from build123d import *

# Parameters (mm, degrees)
SKETCH1_R                 = 13
BOSS_EXTRUDE1_DEPTH       = 65
BOSS_EXTRUDE1_DEPTH_BACK  = 65
SKETCH6_R                 = 2.5
BOSS_EXTRUDE5_DEPTH       = 35
SKETCH7_R                 = 2.5
BOSS_EXTRUDE6_DEPTH       = 35
SKETCH10_R                = 2.5
BOSS_EXTRUDE7_DEPTH       = 20
BOSS_EXTRUDE7_DEPTH_BACK  = 20
SKETCH11_R                = 2.5
BOSS_EXTRUDE8_DEPTH       = 45
SKETCH12_W                = 11.53
SKETCH12_H                = 5
BOSS_EXTRUDE9_DEPTH       = 12
SKETCH13_R                = 4.765
CUT_EXTRUDE2_DEPTH        = 66
CUT_EXTRUDE2_DEPTH_BACK   = 12
SKETCH14_R                = 2.5
BOSS_EXTRUDE10_DEPTH      = 20
BOSS_EXTRUDE10_DEPTH_BACK = 20
SKETCH15_R                = 2.5
BOSS_EXTRUDE11_DEPTH      = 45
SKETCH16_W                = 11.53
SKETCH16_H                = 5
BOSS_EXTRUDE12_DEPTH      = 12
SKETCH17_R                = 4.765
CUT_EXTRUDE3_DEPTH        = 12
CUT_EXTRUDE3_DEPTH_BACK   = 51


with BuildPart() as part:
    # Sketch1 → Boss-Extrude1 (new body, two sides)
    with BuildSketch(Plane(origin=(0, 0, 0), x_dir=(0, 0, -1), z_dir=(1, 0, 0))) as boss_extrude1_sk:
        Circle(SKETCH1_R)
    extrude(amount=BOSS_EXTRUDE1_DEPTH)
    extrude(boss_extrude1_sk.sketch, amount=-BOSS_EXTRUDE1_DEPTH_BACK)

    # Sketch6 → Boss-Extrude5 (add)
    with BuildSketch(Plane(origin=(65, 0, 0), x_dir=(0, 0, -1), z_dir=(1, 0, 0))):
        Circle(SKETCH6_R)
    extrude(amount=BOSS_EXTRUDE5_DEPTH)

    # Sketch7 → Boss-Extrude6 (add)
    with BuildSketch(Plane.ZY.offset(65)):
        Circle(SKETCH7_R)
    extrude(amount=BOSS_EXTRUDE6_DEPTH)

    # Sketch10 → Boss-Extrude7 (add, two sides)
    with BuildSketch(Plane.YX) as boss_extrude7_sk:
        with Locations((0, 100)):
            Circle(SKETCH10_R)
    extrude(amount=BOSS_EXTRUDE7_DEPTH)
    extrude(boss_extrude7_sk.sketch, amount=-BOSS_EXTRUDE7_DEPTH_BACK)

    # Sketch11 → Boss-Extrude8 (add)
    with BuildSketch(Plane(origin=(0, 0, 0), x_dir=(1, 0, 0), z_dir=(0, 1, 0))):
        with Locations((100, -20)):
            Circle(SKETCH11_R)
        with Locations((100, 20)):
            Circle(SKETCH11_R)
    extrude(amount=BOSS_EXTRUDE8_DEPTH)

    # Sketch12 → Boss-Extrude9 (add)
    with BuildSketch(Plane(origin=(0, 45, 0), x_dir=(1, 0, 0), z_dir=(0, 1, 0))):
        with Locations((100, -20)):
            Rectangle(SKETCH12_W, SKETCH12_H)
        with Locations((100, 20)):
            Rectangle(SKETCH12_W, SKETCH12_H)
    extrude(amount=BOSS_EXTRUDE9_DEPTH)

    # Sketch13 → Cut-Extrude2 (cut, two sides)
    with BuildSketch(Plane.XY.offset(-17.5)) as cut_extrude2_sk:
        with Locations((100.265, 51)):
            Circle(SKETCH13_R)
    extrude(amount=CUT_EXTRUDE2_DEPTH, mode=Mode.SUBTRACT)
    extrude(cut_extrude2_sk.sketch, amount=-CUT_EXTRUDE2_DEPTH_BACK, mode=Mode.SUBTRACT)

    # Sketch14 → Boss-Extrude10 (add, two sides)
    with BuildSketch(Plane.XY) as boss_extrude10_sk:
        with Locations((-100, 0)):
            Circle(SKETCH14_R)
    extrude(amount=BOSS_EXTRUDE10_DEPTH)
    extrude(boss_extrude10_sk.sketch, amount=-BOSS_EXTRUDE10_DEPTH_BACK)

    # Sketch15 → Boss-Extrude11 (add)
    with BuildSketch(Plane(origin=(0, 0, 0), x_dir=(1, 0, 0), z_dir=(0, 1, 0))):
        with Locations((-100, 20)):
            Circle(SKETCH15_R)
        with Locations((-100, -20)):
            Circle(SKETCH15_R)
    extrude(amount=BOSS_EXTRUDE11_DEPTH)

    # Sketch16 → Boss-Extrude12 (add)
    with BuildSketch(Plane(origin=(0, 45, 0), x_dir=(1, 0, 0), z_dir=(0, 1, 0))):
        with Locations((-100, -20)):
            Rectangle(SKETCH16_W, SKETCH16_H)
        with Locations((-100, 20)):
            Rectangle(SKETCH16_W, SKETCH16_H)
    extrude(amount=BOSS_EXTRUDE12_DEPTH)

    # Sketch17 → Cut-Extrude3 (cut, two sides)
    with BuildSketch(Plane.XY.offset(22.5)) as cut_extrude3_sk:
        with Locations((-99.735, 51)):
            Circle(SKETCH17_R)
    extrude(amount=CUT_EXTRUDE3_DEPTH, mode=Mode.SUBTRACT)
    extrude(cut_extrude3_sk.sketch, amount=-CUT_EXTRUDE3_DEPTH_BACK, mode=Mode.SUBTRACT)


solid = part.part
The model under review builds one solid part; all positions refer to its coordinate system, in mm. A direction names the side the tool comes from. Give positions to 0.01 mm unless a question says otherwise; leave off trailing zeros. Order: outer loops, then holes, each group sorted by start corner. A loop starts at its lowest first (then second) coordinate and runs counter-clockwise, first axis right, second up. Notation, with made-up numbers: (33.5, -34.75) -> (38.5, -34.75) arc R17 cw to (38.5, -3.75) -> close; hole circle Ø1 at (-25, 26.25). An arc over 180 degrees is marked (long way). Write item = value, one per line. Start each with the question number.
(1) Draft analysis for pull direction X (two halves, no side actions). For faces 1 (the flat face through (-104, 54, 22.5)), 2 (the flat face through (105.765, 51, -20)), 3 (the cylindrical face through (-104.495, 51.21, 20.035)), state which applies: +X half, -X half, draft (parallel to the pull), parting line (faces both ways), or undercut.
(2) Tool access review of faces 4 (the flat face through (-94.235, 51, -20)), 5 (the flat face through (-105.765, 51, 20)), 6 (the cylindrical face through (82.3, 0.1, 2.5)), 7 (the flat face through (-104, 54, -22.5)), 8 (the flat face through (96, 54, -17.5)): name each direction out of +Z, -Z, +X, -X, +Y, -Y from which nothing blocks a thin tool from reaching the whole face with its end or side.
(3) For pin 1 Ø1 at (x, z) = (-66, 9.5) entering from +Y; pin 2 Ø1.5 at (x, z) = (97, -19) entering from -Y; pin 3 Ø1.5 at (x, z) = (-101.5, 21) entering from -Y; pin 4 Ø2.5 at (x, z) = (97.5, 19) entering from -Y, all flat-tipped, find the tip position at first contact; note any pin that passes through.
(4) Take a section at A-A (y = 51). State how many separate pieces and enclosed holes the cut face has, plus the area to 3 significant figures.
(5) For L1, parallel to X at y = 44, z = -19; L2, parallel to Z at x = 75, y = 1.5; L3, parallel to Y at x = -56, z = 3, list the stretches that pass through material, from the lowest coordinate up. Write a range as from..to.
(6) Take a section at D-D (z = 15.5). Write out the cut boundary in (x, y), plus the area to 3 significant figures.
(7) Take a section at C-C (y = 18.5). Write out the cut boundary in (x, z), plus the area to 3 significant figures.
(8) Take a section at B-B (z = 0). Write out the cut boundary in (x, y), plus the area to 3 significant figures.
Returned:
q1.face_1 = draft
q1.face_2 = +X half
q1.face_3 = undercut
q2.face_4 = +Z, -Z, +Y, -Y
q2.face_5 = +Z, -Z, -X, +Y, -Y
q2.face_6 = none
q2.face_7 = -Z, +X, -X, +Y, -Y
q2.face_8 = +X, -X, +Y
q3.pin_1 = through
q3.pin_2 = -1.09
q3.pin_3 = 0
q3.pin_4 = -2.17
q4.separate_pieces = 8
q4.enclosed_holes = 0
q4.area = 40.0 mm²
q5.L1 = -102.29..-97.71, 97.71..102.29
q5.L2 = -2..2
q5.L3 = -12.65..12.65
q6.outline = circle Ø5 at (-100, 0); circle Ø5 at (100, 0)
q6.area = 39.3 mm²
q7.outline = circle Ø5 at (-100, -20); circle Ø5 at (-100, 20); circle Ø5 at (100, -20); circle Ø5 at (100, 20)
q7.area = 78.5 mm²
q8.outline = (-100, -2.5) -> (-65, -2.5) -> (-65, -13) -> (65, -13) -> (65, -2.5) -> (100, -2.5) arc R2.5 ccw to (100, 2.5) -> (65, 2.5) -> (65, 13) -> (-65, 13) -> (-65, 2.5) -> (-100, 2.5) arc R2.5 ccw to start
q8.area = 3,750 mm²
